```python
from build123d import *

# Parameters (mm, degrees)
SKETCH2_W                  = 20.32
SKETCH2_H                  = 2.41
BOSS_EXTRUDE1_DEPTH        = 8.51
SKETCH5_W                  = 1
SKETCH5_H                  = 1
CUT_EXTRUDE1_DEPTH         = 5
CHAMFER1_SIZE              = 0.5
LPATTERN3_COUNT            = 8
LPATTERN3_PITCH            = 2.54
CHAMFER1_OF_LPATTERN3_SIZE = 0.5
BOSS_EXTRUDE2_DEPTH        = 11
LPATTERN1_COUNT            = 8
LPATTERN1_PITCH            = 2.54


with BuildPart() as part:
    # Sketch2 → Boss-Extrude1 (new body)
    with BuildSketch(Plane(origin=(0, 0, 0), x_dir=(1, 0, 0), z_dir=(0, 1, 0))):
        with Locations((8.89, 0)):
            Rectangle(SKETCH2_W, SKETCH2_H)
    extrude(amount=BOSS_EXTRUDE1_DEPTH)

    # Sketch5 → Cut-Extrude1 (cut)
    with BuildSketch(Plane(origin=(0, 8.51, 0), x_dir=(1, 0, 0), z_dir=(0, 1, 0))):
        Rectangle(SKETCH5_W, SKETCH5_H)
    cut_extrude1 = extrude(amount=-CUT_EXTRUDE1_DEPTH, mode=Mode.SUBTRACT)

    # Chamfer1
    chamfer1_edges = [part.edges().sort_by_distance(p)[0] for p in [
        (0.5, 8.51, 0),
        (0, 8.51, -0.5),
        (-0.5, 8.51, 0),
        (0, 8.51, 0.5),
    ]]
    chamfer(chamfer1_edges, length=CHAMFER1_SIZE)

    # LPattern3: Cut-Extrude1 ×8
    with Locations(*[(i * LPATTERN3_PITCH, 0, 0) for i in range(1, LPATTERN3_COUNT)]):
        add(cut_extrude1, mode=Mode.SUBTRACT)

    # Chamfer1 of LPattern3
    chamfer1_of_lpattern3_edges = [part.edges().sort_by_distance(p)[0] for p in [
        (3.04, 8.51, 0),
        (2.54, 8.51, -0.5),
        (2.04, 8.51, 0),
        (2.54, 8.51, 0.5),
        (5.58, 8.51, 0),
        (5.08, 8.51, -0.5),
        (4.58, 8.51, 0),
        (5.08, 8.51, 0.5),
        (8.12, 8.51, 0),
        (7.62, 8.51, -0.5),
        (7.12, 8.51, 0),
        (7.62, 8.51, 0.5),
        (10.66, 8.51, 0),
        (10.16, 8.51, -0.5),
        (9.66, 8.51, 0),
        (10.16, 8.51, 0.5),
        (13.2, 8.51, 0),
        (12.7, 8.51, -0.5),
        (12.2, 8.51, 0),
        (12.7, 8.51, 0.5),
        (15.74, 8.51, 0),
        (15.24, 8.51, -0.5),
        (14.74, 8.51, 0),
        (15.24, 8.51, 0.5),
        (18.28, 8.51, 0),
        (17.78, 8.51, -0.5),
        (17.28, 8.51, 0),
        (17.78, 8.51, 0.5),
    ]]
    chamfer(chamfer1_of_lpattern3_edges, length=CHAMFER1_OF_LPATTERN3_SIZE)

    # Sketch8 → Boss-Extrude2 (add)
    with BuildSketch(Plane(origin=(0, 0, 0), x_dir=(1, 0, 0), z_dir=(0, 1, 0))):
        with BuildLine():
            Line((-0.3, -0.2), (0.3, -0.2))
            ThreePointArc((0.3, -0.2), (0.370710678, -0.170710678), (0.4, -0.1))
            Line((0.4, -0.1), (0.4, 0.1))
            ThreePointArc((0.4, 0.1), (0.370710678, 0.170710678), (0.3, 0.2))
            Line((0.3, 0.2), (-0.3, 0.2))
            ThreePointArc((-0.3, 0.2), (-0.370710678, 0.170710678), (-0.4, 0.1))
            Line((-0.4, 0.1), (-0.4, -0.1))
            ThreePointArc((-0.4, -0.1), (-0.370710678, -0.170710678), (-0.3, -0.2))
        make_face()
    boss_extrude2 = extrude(amount=-BOSS_EXTRUDE2_DEPTH)

    # LPattern1: Boss-Extrude2 ×8
    with Locations(*[(i * LPATTERN1_PITCH, 0, 0) for i in range(1, LPATTERN1_COUNT)]):
        add(boss_extrude2)


solid = part.part
```
Geometry: final body of the model. Coordinates: model frame, mm. Give positions to 0.01 mm unless a question says otherwise; leave off trailing zeros.
1. Pin query (flat end, axial travel): P1, Ø0.5, axis at x = 10, y = -6, coming from the -Z side. Return the tip coordinate at first contact, or that it passes through.
2. Draft query along Z for faces 1 (the flat face through (9, 0, 0)), 2 (the flat face through (9, 4, 1.205)), 3 (the flat face through (18, 6, -0.5)). Return one class per face: released by +Z, released by -Z, zero draft, split by the parting line, or undercut.
3. Line query: probe 1 along Z at (x, y) = (2.25, 4.5) (3 decimals); probe 2 along Z at (x, y) = (5.25, -2.75); probe 3 along Y at (x, z) = (13, 0.25). Output: solid intervals per line, ascending.
4. Section query A-A, the plane y = 6.75. Count the separate pieces of the cut face and the enclosed holes in it, then the cut area to 3 significant figures.
Computed:
1. P1: stops at z = -0.2
2. face 1: zero draft
2. face 2: released by +Z
2. face 3: undercut
3. probe 1: z = -1.205 to -0.5, 0.5 to 1.205
3. probe 2: z = -0.2 to 0.2
3. probe 3: y = 0 to 3.51
4. separate pieces: 1
4. enclosed holes: 8
4. area: 41.0 mm2
